For this review, take the finished solid that the model builds, in its own axes (mm). Face numbers are marked on the shaded views. A direction names the side the tool comes from. Give positions to 0.01 mm unless a question says otherwise; leave off trailing zeros. Loops run counter-clockwise (first coordinate to the right, second up) from the corner with the lowest first, then second, coordinate; pieces in that order, holes last. Notation, with made-up numbers: (5, 15.25) - (12, 15.25) arc R6 cw to (12, 20.25) - close; hole circle Ø10 at (4.25, 78.5). An arc over 180 degrees is marked (long way). Put each result on its own line as item: value.
from build123d import *

# Parameters (mm, degrees)
BOSS_EXTRUDE1_DEPTH = 4
BOSS_EXTRUDE2_START = 2
BOSS_EXTRUDE2_DEPTH = 1
SKETCH2_R           = 0.35
BOSS_EXTRUDE3_DEPTH = 1.5
SKETCH3_R           = 0.75
SKETCH3_R_2         = 1.25
CUT_EXTRUDE1_DEPTH  = 0.01


with BuildPart() as part:
    # Sketch1 → Boss-Extrude1 (new body)
    with BuildSketch(Plane(origin=(0, 0, 0), x_dir=(1, 0, 0), z_dir=(0, 1, 0))):
        with BuildLine():
            Line((4.25, 2), (-4.25, 2))
            ThreePointArc((-4.25, 2), (-6.25, 0), (-4.25, -2))
            Line((-4.25, -2), (4.25, -2))
            ThreePointArc((4.25, -2), (6.25, 0), (4.25, 2))
        make_face()
    extrude(amount=BOSS_EXTRUDE1_DEPTH)

    # Sketch1<3> → Boss-Extrude2 (add)
    with BuildSketch(Plane(origin=(0, 0, 0), x_dir=(1, 0, 0), z_dir=(0, 1, 0)).offset(BOSS_EXTRUDE2_START)):
        with BuildLine():
            Line((5.25, 2), (4.25, 2))
            ThreePointArc((4.25, 2), (6.25, 0), (4.25, -2))
            Line((4.25, -2), (5.25, -2))
            ThreePointArc((5.25, -2), (7.25, 0), (5.25, 2))
        make_face()
        with BuildLine():
            Line((-4.25, 2), (-5.25, 2))
            ThreePointArc((-5.25, 2), (-7.25, 0), (-5.25, -2))
            Line((-5.25, -2), (-4.25, -2))
            ThreePointArc((-4.25, -2), (-6.25, 0), (-4.25, 2))
        make_face()
    extrude(amount=BOSS_EXTRUDE2_DEPTH)

    # Sketch2 → Boss-Extrude3 (add)
    with BuildSketch(Plane(origin=(0, 4, 0), x_dir=(1, 0, 0), z_dir=(0, 1, 0))):
        with Locations((-1.25, 0)):
            Circle(SKETCH2_R)
        with Locations((1.25, 0)):
            Circle(SKETCH2_R)
    extrude(amount=BOSS_EXTRUDE3_DEPTH)

    # Sketch3 → Cut-Extrude1 (cut)
    with BuildSketch(Plane.XZ):
        with Locations((-1.25, 0)):
            Circle(SKETCH3_R)
        with Locations((1.25, 0)):
            Circle(SKETCH3_R)
        with Locations((4.25, 0)):
            Circle(SKETCH3_R_2)
        with Locations((-4.25, 0)):
            Circle(SKETCH3_R_2)
    extrude(amount=-CUT_EXTRUDE1_DEPTH, mode=Mode.SUBTRACT)


solid = part.part
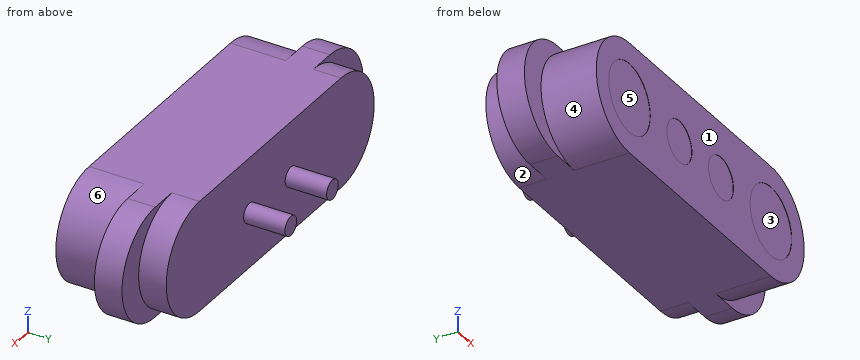
1) Take a section at B-B on z = 1.4. State the section outline as (x, y) points, and give its area (3 significant figures).
Geometry check:
outline: (-6.68, 2) - (-5.68, 2) - (-5.68, 0) - (5.68, 0) - (5.68, 2) - (6.68, 2) - (6.68, 3) - (5.68, 3) - (5.68, 4) - (-5.68, 4) - (-5.68, 3) - (-6.68, 3) - close
area: 47.4 mm²
2) Insertion check: pin 1 Ø1.5 at (x, z) = (6.5, 0) entering from +Y; pin 2 Ø1.5 at (x, z) = (-4.25, 0) entering from -Y. Each pin has a flat end and moves straight along its axis. Give the tip position at first contact, or say it passes through.
Geometry check:
pin 1: stops at y = 4
pin 2: stops at y = 0.01
3) Wall thickness on line 1 (Y direction, x = 6, z = 0.3); line 2 (X direction, y = 0.45, z = 0.1); line 3 (Y direction, x = 6.75, z = 0.35): over which ranges is each line inside the solid? List them lowest first.
Geometry check:
line 1: y = 0 to 4
line 2: x = -6.25 to 6.25
line 3: y = 2 to 3
4) Take a section at C-C on y = 0.75. State the section outline as (x, z) points, and give its area (3 significant figures).
Geometry check:
outline: (-4.25, -2) - (4.25, -2) arc R2 ccw to (4.25, 2) - (-4.25, 2) arc R2 ccw to start
area: 46.6 mm²
5) Draft analysis for pull direction X (two halves, no side actions). For the marked faces 1, 2 and 3, state which applies: pulls with the +X half, pulls with the -X half, needs draft (parallel to the pull), parting line crosses it, or undercut.
Geometry check:
face 1: needs draft
face 2: pulls with the -X half
face 3: undercut
6) For the marked faces 4, 5 and 6, list the 3-axis set-ups (+Z, -Z, +X, -X, +Y, -Y) from which the entire face can be reached by the end or side of a thin tool; tool diameter is ignored.
Geometry check:
face 4: -X, -Y
face 5: -Y
face 6: +X, -Y
